Part model, mm, in its own coordinate system. Face numbers are marked on the shaded views. A direction names the side the tool comes from. Give positions to 0.01 mm unless a question says otherwise; leave off trailing zeros. Order: outer loops, then holes, each group sorted by start corner. A loop starts at its lowest first (then second) coordinate and runs counter-clockwise, first axis right, second up. Notation, with made-up numbers: (52.5, -3) - (62.5, -3) arc R28 cw to (62.5, 18) - close; hole circle Ø1 at (-13.75, 41.25). An arc over 180 degrees is marked (long way). Use one line per item in the form item = value. Start each with the question number.
1. Band-saw the part on D-D, the plane x = 10.5. List the corners of the cut face in (y, z).
2. Band-saw the part on C-C, the plane z = 13.5. List the corners of the cut face in (x, y), plus the area to 3 significant figures.
3. Pull direction Z, two halves, no side cores. Call the marked faces 1, 2 and 3: +Z half, -Z half, draft (parallel to the pull), parting line (faces both ways), or undercut.
4. Pin check, flat tips, straight feed: P1, Ø1.5, axis at y = 40.5, z = -9.5, coming from the -X side; P2, Ø1.5, axis at x = 56, z = -9.5, coming from the +Y side; P3, Ø5, axis at y = 17.5, z = -6, coming from the -X side. Stop position of each tip, or through.
5. Band-saw the part on A-A, the plane x = 68. List the corners of the cut face in (y, z), plus the area to 3 significant figures.
6. Band-saw the part on B-B, the plane y = 33.5. List the corners of the cut face in (x, z), plus the area to 3 significant figures.
7. Drill centre lines: line 1 (Y direction, x = 78.5, z = -13); line 2 (X direction, y = 3, z = -11); line 3 (Z direction, x = 13.5, y = 16). Where is each one in solid material? Low to high.
8. Tool access for the marked faces 4, 5, 6, 7 and 8: list every direction of +Z, -Z, +X, -X, +Y, -Y with a clear straight run to the whole face (end or side of a thin tool).
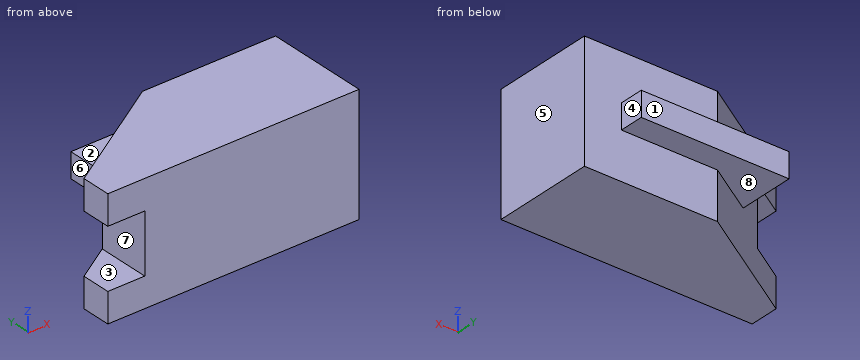
from build123d import *

# Parameters (mm, degrees)
BOSS_EXTRUDE1_DEPTH = 24
SKETCH2_W           = 60
SKETCH2_H           = 10
BOSS_EXTRUDE2_DEPTH = 52
CUT_EXTRUDE1_REACH  = 118.979
SKETCH3_W           = 15
SKETCH3_H           = 24


with BuildPart() as part:
    # Sketch1 → Boss-Extrude1 (new, symmetric)
    with BuildSketch(Plane.XY):
        Polygon((0, 0), (102, 0), (102, 42), (48, 42), (0, 12), align=None)
    extrude(amount=BOSS_EXTRUDE1_DEPTH, both=True)

    # Sketch2 → Boss-Extrude2 (add)
    with BuildSketch(Plane(origin=(0, 0, 0), x_dir=(1, 0, 0), z_dir=(0, 1, 0))):
        with Locations((57, 0)):
            Rectangle(SKETCH2_W, SKETCH2_H)
    extrude(amount=BOSS_EXTRUDE2_DEPTH)

    # Cut-Extrude1: up to this plane
    cut_extrude1_end = Plane(origin=(48, 42, 24), z_dir=(0.52999894000318, -0.8479983040050879, 0))
    # Sketch3 → Cut-Extrude1 (cut, up to the surface)
    with BuildSketch(Plane(origin=(0, 0, 0), x_dir=(1, 0, 0), z_dir=(0, 1, 0)), mode=Mode.PRIVATE) as cut_extrude1_sk1:
        with Locations((7.5, 0)):
            Rectangle(SKETCH3_W, SKETCH3_H)
    cut_extrude1_tool1 = split(extrude(cut_extrude1_sk1.sketch, amount=CUT_EXTRUDE1_REACH, mode=Mode.PRIVATE), bisect_by=cut_extrude1_end, keep=Keep.BOTH, mode=Mode.PRIVATE)
    add(cut_extrude1_tool1.solids().sort_by_distance((7.5, 0, 0))[0], mode=Mode.SUBTRACT)


solid = part.part
From the geometry:
q1.outline = (0, -24) - (18.56, -24) - (18.56, -12) - (0, -12) - close; (0, 12) - (18.56, 12) - (18.56, 24) - (0, 24) - close
q2.outline = (0, 0) - (102, 0) - (102, 42) - (48, 42) - (0, 12) - close
q2.area = 3,560 mm²
q3.face_1 = draft
q3.face_2 = +Z half
q3.face_3 = undercut
q4.P1 = 44.4
q4.P2 = 42
q4.P3 = 15
q5.outline = (0, -24) - (42, -24) - (42, -5) - (52, -5) - (52, 5) - (42, 5) - (42, 24) - (0, 24) - close
q5.area = 2,120 mm²
q6.outline = (27, -5) - (34.4, -5) - (34.4, -24) - (102, -24) - (102, 24) - (34.4, 24) - (34.4, 5) - (27, 5) - close
q6.area = 3,320 mm²
q7.line_1 = 0 to 42
q7.line_2 = 15 to 102
q7.line_3 = -24 to -12, 12 to 24
q8.face_4 = +Z, -Z, +X, +Y
q8.face_5 = +Z, -Z, +X, +Y, -Y
q8.face_6 = +Z, -Z, -X, +Y
q8.face_7 = -X, +Y, -Y
q8.face_8 = -Z, -X, +Y
